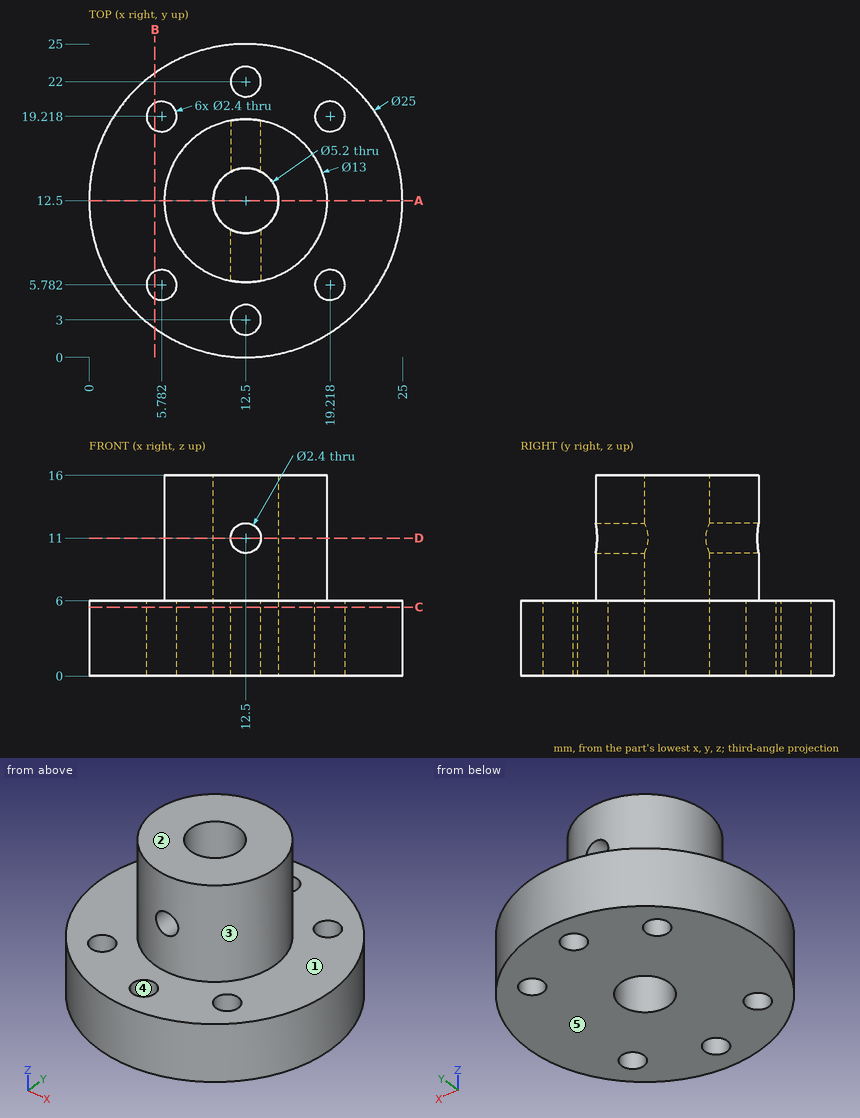
The figure shows three views and two pictorial views of one solid part (mm, origin at its lowest corner). Answer the questions. A direction names the side the tool comes from. Give positions to 0.01 mm unless a question says otherwise; leave off trailing zeros. Order: outer loops, then holes, each group sorted by start corner. A loop starts at its lowest first (then second) coordinate and runs counter-clockwise, first axis right, second up. Notation, with made-up numbers: (-23.5, -37.5) -> (29.5, -37.5) arc R19 cw to (29.5, -21.5) -> close; hole circle Ø5 at (-30, 19.5). An arc over 180 degrees is marked (long way). One line per item, written item: value.
1) Find the intervals of material crossed by line 1 (Z direction, x = 12.5, y = 17.5); line 2 (Y direction, x = 6.5, z = 4) (1 decimal); line 3 (X direction, y = 5.75, z = 4.75) (1 decimal), in increasing order.
Reported:
line 1: z = 0 to 9.8, 12.2 to 16
line 2: y = 1.5 to 4.8, 6.7 to 18.3, 20.2 to 23.5
line 3: x = 2 to 4.6, 7 to 18, 20.4 to 23
2) Find section D-D, the plane z = 11. Determine the outline of the cut face in (x, y).
Reported:
outline: (11.3, 6.11) -> (11.3, 10.19) arc R2.6 cw to (11.3, 14.81) -> (11.3, 18.89) arc R6.5 ccw to start; (13.7, 6.11) arc R6.5 ccw to (13.7, 18.89) -> (13.7, 14.81) arc R2.6 cw to (13.7, 10.19) -> close
3) Find section C-C, the plane z = 5.5. Determine the outline of the cut face in (x, y).
Reported:
outline: circle Ø25 at (12.5, 12.5); hole circle Ø2.4 at (5.78, 5.78); hole circle Ø2.4 at (5.78, 19.22); hole circle Ø5.2 at (12.5, 12.5); hole circle Ø2.4 at (12.5, 3); hole circle Ø2.4 at (12.5, 22); hole circle Ø2.4 at (19.22, 5.78); hole circle Ø2.4 at (19.22, 19.22)
4) Find section A-A, the plane y = 12.5. Determine the outline of the cut face in (x, z), plus the area to 3 significant figures.
Reported:
outline: (0, 0) -> (9.9, 0) -> (9.9, 16) -> (6, 16) -> (6, 6) -> (0, 6) -> close; (15.1, 0) -> (25, 0) -> (25, 6) -> (19, 6) -> (19, 16) -> (15.1, 16) -> close
area: 197 mm^2
5) Flat-ended cylindrical pins translate along their axes: P1, Ø5, axis at x = 6.5, z = 10, coming from the +Y side; P2, Ø7.5, axis at x = 15, y = 13, coming from the +Z side; P3, Ø1, axis at x = 15, z = 7.5, coming from the +Y side (1 decimal); P4, Ø5, axis at x = 9.5, z = 7.5, coming from the +Y side. Find the tip coordinate at first contact, or state that the pin passes through.
Reported:
P1: stops at y = 17.98
P2: stops at z = 16
P3: stops at y = 18.7
P4: stops at y = 24.96
6) Find section B-B, the plane x = 5.25. Determine the outline of the cut face in (y, z).
Reported:
outline: (2.32, 0) -> (4.71, 0) -> (4.71, 6) -> (2.32, 6) -> close; (6.86, 0) -> (18.14, 0) -> (18.14, 6) -> (6.86, 6) -> close; (20.29, 0) -> (22.68, 0) -> (22.68, 6) -> (20.29, 6) -> close
7) A tool of negligible diameter and unlimited length cuts with its end or side. For the marked faces 1 and 2, from which of +Z, -Z, +X, -X, +Y, -Y can it reach the whole face along a straight path? Write none if from no direction.
Reported:
face 1: +Z
face 2: +Z, +X, -X, +Y, -Y
8) Determine the mould class of the marked faces 3, 4 and 5 for opening direction Y: pulls with the +Y half, pulls with the -Y half, needs draft (parallel to the pull), parting line crosses it, or undercut.
Reported:
face 3: parting line crosses it
face 4: undercut
face 5: needs draft
